Build history of the part. All positions in model axes, mm. A direction names the side the tool comes from. Round coordinates to 2 decimals unless told otherwise and drop trailing zeros. Write each loop counter-clockwise with the first axis right and the second up, starting at its lowest first coordinate (ties: lowest second). Pieces come first, ordered by that corner, then holes. Notation, with made-up numbers: M 28,26 L 81,26 A19 cw 81,40 Z; hole C -17.5,39 d6. An arc over 180 degrees is marked long. Write item = value, one per line. Start each with the question number.
Q1. Band-saw the part on A-A on x = 39. Write the cut outline in (y, z).
Q2. Band-saw the part on D-D on y = 82.5. Write the cut outline in (x, z).
Q3. Pull direction X, two halves, no side cores. Call faces 1 (the flat face through (5.954, 12.375, 14.493)), 2 (the flat face through (11, 4.986, 8)), 3 (the flat face through (53.627, 1.345, 0.493)): released by +X, released by -X, zero draft, split by the parting line, or undercut.
Q4. Probe L1, parallel to Y at x = 15, z = 4.5; L2, parallel to X at y = 44, z = 12.5; L3, parallel to X at y = 58.5, z = 7.5. List the from-to ranges inside material, lowest first.
Q5. Band-saw the part on C-C on z = 9.75. Write the cut outline in (x, y) (1 decimal), plus the area to 3 significant figures.
Q6. Tool access for faces 4 (the flat face through (47.25, 63.76, 0.49)), 5 (the flat face through (33.55, 35.184, 14.507)), 6 (the flat face through (53.99, 88.15, 7.59)), 7 (the flat face through (54, 1, 8)), 8 (the flat face through (13.03, 11.22, 7.41)): list every direction of +Z, -Z, +X, -X, +Y, -Y with a clear straight run to the whole face (end or side of a thin tool).
Q7. Band-saw the part on B-B on y = 39. Write the cut outline in (x, z).
Q8. Drop flat-ended pins along their axis: P1, Ø6, axis at x = 22, y = 25, coming from the -Z side; P2, Ø5.5, axis at y = 73.5, z = 6.5, coming from the -X side; P3, Ø9, axis at x = 9.5, z = 7.5, coming from the +Y side; P4, Ø4, axis at x = 39.5, y = 75.5, coming from the +Z side. Give the stop position or say it passes through.
Autodesk Fusion 360 part; units mm, degrees
sketch "Sketch1" plane through (0, 0, 0) normal (0, 0, 1) x (1, 0, 0)
  line L0 (0, 0) -> (5.1303, 14.0954)
  line L1 (0, 0) -> (15, 0) construction
  line L2 (5.1303, 14.0954) -> (19.2257, 8.9651)
  line L3 (5.1303, 14.0954) -> (20.1303, 14.0954) construction
  line L4 (19.2257, 8.9651) -> (46.5873, 84.1405)
  line L5 (19.2257, 8.9651) -> (99.2257, 8.9651) construction
  line L6 (46.5873, 84.1405) -> (55, 84.1405)
  line L7 (55, 84.1405) -> (55, 0)
  line L8 (55, 0) -> (0, 0)
  dimension "d1" = 70
  dimension "d2" = 15
  dimension "d3" = 20
  dimension "d4" = 15
  dimension "d5" = 70
  dimension "d6" = 80
extrude "Extrude1" add sketch "Sketch1" along normal blind 15
sketch "Sketch2" plane through (0, 0, 15) normal (0, 0, 1) x (-1, 0, 0)
  line L0 (-55, 0) -> (-55, -84.1405)
  line L1 (-55, -84.1405) -> (-46.5873, -84.1405)
  line L2 (-46.5873, -84.1405) -> (-19.2257, -8.9651)
  line L3 (-19.2257, -8.9651) -> (-5.1303, -14.0954)
  line L4 (-5.1303, -14.0954) -> (0, 0)
  line L5 (0, 0) -> (-55, 0)
  line L6 (-23.9242, -7.255) -> (-49.9527, -78.7679)
  line L7 (-23.9242, -7.255) -> (52.1783, -7.255) construction
  line L8 (-49.9527, -78.7679) -> (-49.9527, -5)
  line L9 (-23.9242, -7.255) -> (-30.1197, -5)
  line L10 (-23.9242, -7.255) -> (-17.331, -7.255) construction
  line L11 (-49.9527, -5) -> (-30.1197, -5)
  dimension "d13" = 5
  dimension "d14" = 110
  dimension "d15" = 160
extrude "Extrude2" cut sketch "Sketch2" against normal blind 78 contours L6 L8 L9 L11
sketch "Sketch3" plane through (0, 0, 15) normal (0, 0, 1) x (-1, 0, 0)
  line L0 (-49.9527, -5) -> (-30.1197, -5)
  line L1 (-30.1197, -5) -> (-23.9242, -7.255)
  line L2 (-23.9242, -7.255) -> (-49.9527, -78.7679)
  line L3 (-49.9527, -78.7679) -> (-49.9527, -5)
  line L4 (-55, 0) -> (-55, -84.1405)
  line L5 (-55, -84.1405) -> (-46.5873, -84.1405)
  line L6 (-46.5873, -84.1405) -> (-19.2257, -8.9651)
  line L7 (-19.2257, -8.9651) -> (-5.1303, -14.0954)
  line L8 (-5.1303, -14.0954) -> (0, 0)
  line L9 (0, 0) -> (-55, 0)
  line L10 (-7.1358, -4.9864) -> (-15.5382, -4.9864)
  line L11 (-7.1358, -4.9864) -> (-8.1187, -7.6868)
  line L12 (-8.1187, -7.6868) -> (-15.5382, -4.9864)
extrude "Extrude3" cut sketch "Sketch3" against normal blind 57 contours L10 L11 L12
chamfer "Chamfer1" distance 2 angle 45 1 edges at (0, 0, 7.5)
chamfer "Chamfer2" distance 2 angle 45 1 edges at (55, 0, 7.5)
chamfer "Chamfer3" distance 2 angle 45 1 edges at (5.1303, 14.0954, 7.5)
chamfer "Chamfer8" distance 16 angle 45 1 edges at (49.9527, 78.7679, 7.5)
sketch "Sketch4" plane through (0, 0, 15) normal (0, 0, 1) x (-1, 0, 0)
  line L0 (-49.9527, -5) -> (-30.1197, -5)
  line L1 (-30.1197, -5) -> (-23.9242, -7.255)
  line L2 (-23.9242, -7.255) -> (-44.4804, -63.7328)
  line L3 (-44.4804, -63.7328) -> (-49.9527, -62.7679)
  line L4 (-49.9527, -62.7679) -> (-49.9527, -5)
  line L5 (-8.1187, -7.6868) -> (-15.5382, -4.9864)
  line L6 (-15.5382, -4.9864) -> (-7.1358, -4.9864)
  line L7 (-7.1358, -4.9864) -> (-8.1187, -7.6868)
  line L8 (-49.9527, -78.7679) -> (-46.2169, -68.5038)
  line L9 (-49.9527, -78.7679) -> (-49.9527, -67.8451)
  line L10 (-46.2169, -68.5038) -> (-49.9527, -67.8451)
  line L11 (-7.0097, -13.4113) -> (-4.4463, -12.216)
  line L12 (-4.4463, -12.216) -> (-0.684, -1.8794)
  line L13 (-0.684, -1.8794) -> (-2, 0)
  line L14 (-2, 0) -> (-53, 0)
  line L15 (-53, 0) -> (-55, -2)
  line L16 (-55, -2) -> (-55, -84.1405)
  line L17 (-55, -84.1405) -> (-46.5873, -84.1405)
  line L18 (-46.5873, -84.1405) -> (-19.2257, -8.9651)
  line L19 (-19.2257, -8.9651) -> (-7.0097, -13.4113)
extrude "Extrude4" cut sketch "Sketch4" against normal blind 36 contours L8 L9 L10
chamfer "Chamfer9" distance 1 angle 45 5 edges at (34.2023, 35.4939, 15) (27.0219, 6.1275, 15) (40.0362, 5, 15) (49.9527, 33.884, 15) (47.2166, 63.2504, 15)
chamfer "Chamfer10" distance 1 angle 45 5 edges at (49.9527, 33.884, 0) (47.2166, 63.2504, 0) (34.2023, 35.4939, 0) (27.0219, 6.1275, 0) (40.0362, 5, 0)
chamfer "Chamfer11" distance 1 angle 45 3 edges at (11.337, 4.9864, 15) (11.8284, 6.3366, 15) (7.6272, 6.3366, 15)
extrude "Extrude5" add 1 faces at (49.3915, 84.1405, 5) along direction (0, 1, 0) blind 5
sketch "Sketch5" plane through (0, 0, 15) normal (0, 0, 1) x (-1, 0, 0)
  line L0 (-50.9527, -63.607) -> (-50.9527, -4)
  line L1 (-50.9527, -4) -> (-29.9434, -4)
  line L2 (-29.9434, -4) -> (-22.6424, -6.6573)
  line L3 (-22.6424, -6.6573) -> (-43.8277, -64.8634)
  line L4 (-43.8277, -64.8634) -> (-50.9527, -63.607)
  line L5 (-49.9527, -67.8451) -> (-46.2169, -68.5038)
  line L6 (-46.2169, -68.5038) -> (-49.9527, -78.7679)
  line L7 (-49.9527, -78.7679) -> (-49.9527, -67.8451)
  line L8 (-7.0097, -13.4113) -> (-4.4463, -12.216)
  line L9 (-4.4463, -12.216) -> (-0.684, -1.8794)
  line L10 (-0.684, -1.8794) -> (-2, 0)
  line L11 (-2, 0) -> (-53, 0)
  line L12 (-53, 0) -> (-55, -2)
  line L13 (-55, -2) -> (-55, -89.1405)
  line L14 (-55, -89.1405) -> (-46.5873, -89.1405)
  line L15 (-46.5873, -89.1405) -> (-46.5873, -84.1405)
  line L16 (-46.5873, -84.1405) -> (-19.2257, -8.9651)
  line L17 (-19.2257, -8.9651) -> (-7.0097, -13.4113)
  line L18 (-5.7076, -3.9864) -> (-7.521, -8.9685)
  line L19 (-7.521, -8.9685) -> (-21.2094, -3.9864)
  line L20 (-21.2094, -3.9864) -> (-5.7076, -3.9864)
  line L21 (-46.5873, -84.1405) -> (-48.4072, -89.1405)
  line L22 (-46.5873, -84.1405) -> (-41.2664, -84.1405) construction
  dimension "d43" = 110
extrude "Extrude6" cut sketch "Sketch5" against normal blind 20 contours L14 L15 L21
chamfer "Chamfer12" distance 1 angle 45 3 edges at (48.0848, 73.6359, 15) (49.9527, 73.3065, 15) (48.0848, 68.1744, 15)
chamfer "Chamfer13" distance 2 angle 45 2 edges at (48.4072, 89.1405, 7.5) (55, 89.1405, 7.5)
chamfer "Chamfer14" distance 1 angle 45 11 edges at (5.728, 12.8137, 15) (2.5652, 7.0477, 15) (1.342, 0.9397, 15) (27.5, 0, 15) (13.1177, 11.1882, 15) (33.4744, 48.1131, 15) (55, 44.5702, 15) (54, 1, 15) (54, 88.1405, 15) (51.7036, 89.1405, 15) (49.0651, 88.2008, 15)
chamfer "Chamfer15" distance 1 angle 45 11 edges at (55, 44.5702, 0) (54, 88.1405, 0) (51.7036, 89.1405, 0) (49.0651, 88.2008, 0) (33.4744, 48.1131, 0) (13.1177, 11.1882, 0) (5.728, 12.8137, 0) (2.5652, 7.0477, 0) (1.342, 0.9397, 0) (27.5, 0, 0) (54, 1, 0)
chamfer "Chamfer16" distance 1 angle 45 3 edges at (49.9527, 73.3065, 0) (48.0848, 73.6359, 0) (48.0848, 68.1744, 0)
chamfer "Chamfer17" distance 1 angle 45 3 edges at (11.337, 4.9864, 0) (11.8284, 6.3366, 0) (7.6272, 6.3366, 0)
Conclusion:
q1.outline = M 0,1 L 1,0 L 4,0 L 5,1 L 5,14 L 4,15 L 1,15 L 0,14 Z; M 48.68,1 L 51.6,0 L 60.37,0 L 63.29,1 L 63.29,14 L 60.37,15 L 51.6,15 L 48.68,14 Z
q2.outline = M 45.99,1 L 47.05,0 L 50.25,0 L 50.61,0.34 L 50.95,0 L 54,0 L 55,1 L 55,14 L 54,15 L 50.95,15 L 50.61,14.66 L 50.25,15 L 47.05,15 L 45.99,14 Z
q3.face_1 = released by -X
q3.face_2 = undercut
q3.face_3 = released by +X
q4.L1 = 0 to 4.99, 5.18 to 10.5
q4.L2 = 31.98 to 37.3, 49.95 to 55
q4.L3 = 37.25 to 42.58, 49.95 to 55
q5.outline = M 0.7,1.9 L 2,0 L 53,0 L 55,2 L 55,87.1 L 53,89.1 L 50.4,89.1 L 47.7,87.3 L 46.6,84.1 L 19.2,9 L 7,13.4 L 4.4,12.2 Z; hole M 7.1,5 L 15.5,5 L 8.1,7.7 Z; hole M 23.9,7.3 L 30.1,5 L 50,5 L 50,62.8 L 44.5,63.7 Z; hole M 46.2,68.5 L 50,67.8 L 50,78.8 Z
q5.area = 1,240 mm^2
q6.face_4 = -Z
q6.face_5 = +Z
q6.face_6 = +Z, -Z, +X, +Y
q6.face_7 = +Z, -Z, +X, -Y
q6.face_8 = +Z, -Z, +Y
q7.outline = M 30.16,1 L 31.22,0 L 34.41,0 L 35.48,1 L 35.48,14 L 34.41,15 L 31.22,15 L 30.16,14 Z; M 49.95,1 L 50.95,0 L 54,0 L 55,1 L 55,14 L 54,15 L 50.95,15 L 49.95,14 Z
q8.P1 = 0.88
q8.P2 = 41.71
q8.P3 = 13.41
q8.P4 = through
